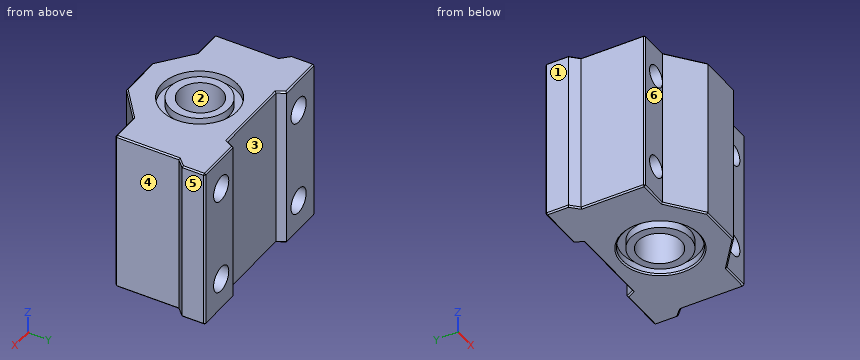
from build123d import *

# Parameters (mm, degrees)
SALIENTE_EXTRUIR1_DEPTH    = 15
CROQUIS2_R                 = 4
CORTAR_EXTRUIR1_DEPTH      = 37.239791666
CORTAR_EXTRUIR2_DEPTH      = 32.800786154
CORTAR_EXTRUIR2_DEPTH_BACK = 32.800786154
CROQUIS3_R                 = 2
SALIENTE_EXTRUIR2_DEPTH    = 30
CROQUIS5_R                 = 7
CROQUIS5_R_2               = 5.5
CORTAR_EXTRUIR3_DEPTH      = 1.5
CORTAR_EXTRUIR4_START      = -1.5
CROQUIS6_R                 = 7
CROQUIS6_R_2               = 5.5
CORTAR_EXTRUIR4_DEPTH      = 1.5
CROQUIS7_R                 = 2.35
CORTAR_EXTRUIR5_DEPTH      = 8.5
CHAFL_N1_SIZE              = 0.25


with BuildPart() as part:
    # Croquis1 → Saliente-Extruir1 (new, symmetric)
    with BuildSketch(Plane.XY):
        Polygon((-4, -11.15), (4, -11.15), (10, -6.35), (15.5, -6.35), (15.5, 5.4), (17, 6.9), (17, 11.15), (10, 11.15), (7.5, 9.65), (-7.5, 9.65), (-10, 11.15), (-17, 11.15), (-17, 6.9), (-15.5, 5.4), (-15.5, -6.35), (-10, -6.35), align=None)
    extrude(amount=SALIENTE_EXTRUIR1_DEPTH, both=True)

    # Croquis2 → Cortar-Extruir1 (cut, through all)
    with BuildSketch(Plane.XY.offset(15)):
        with Locations((0, 0.15)):
            Circle(CROQUIS2_R)
    extrude(amount=-CORTAR_EXTRUIR1_DEPTH, mode=Mode.SUBTRACT)

    # Croquis3 → Cortar-Extruir2 (cut, two sides: drawn at the far end of the back side and taken through both)
    with BuildSketch(Plane(origin=(0, 11.15, 0), x_dir=(1, 0, 0), z_dir=(0, 1, 0)).offset(-CORTAR_EXTRUIR2_DEPTH_BACK)):
        with Locations((-12, 9)):
            Circle(CROQUIS3_R)
        with Locations(Location((12, 9, 0), (0, 0, 180))):
            Circle(CROQUIS3_R)
        with Locations((-12, -9)):
            Circle(CROQUIS3_R)
        with Locations(Location((12, -9, 0), (0, 0, 180))):
            Circle(CROQUIS3_R)
    extrude(amount=CORTAR_EXTRUIR2_DEPTH + CORTAR_EXTRUIR2_DEPTH_BACK, mode=Mode.SUBTRACT)

    # Croquis4 → Saliente-Extruir2 (add, through all)
    with BuildSketch(Plane.XY.offset(15)):
        Polygon((-10, 11.15), (-7.5, 9.65), (-8.3, 11.15), align=None)
        Polygon((7.5, 9.65), (10, 11.15), (8.3, 11.15), align=None)
    extrude(amount=-SALIENTE_EXTRUIR2_DEPTH)

    # Croquis5 → Cortar-Extruir3 (cut)
    with BuildSketch(Plane.XY.offset(15)):
        Circle(CROQUIS5_R)
        Circle(CROQUIS5_R_2, mode=Mode.SUBTRACT)
    extrude(amount=-CORTAR_EXTRUIR3_DEPTH, mode=Mode.SUBTRACT)

    # Croquis6 → Cortar-Extruir4 (cut)
    with BuildSketch(Plane(origin=(0, 0, -15), x_dir=(-1, 0, 0), z_dir=(0, 0, -1)).offset(CORTAR_EXTRUIR4_START)):
        with Locations(Location((0, 0, 0), (0, 0, 180))):
            Circle(CROQUIS6_R)
        with Locations(Location((0, 0, 0), (0, 0, 180))):
            Circle(CROQUIS6_R_2, mode=Mode.SUBTRACT)
    extrude(amount=CORTAR_EXTRUIR4_DEPTH, mode=Mode.SUBTRACT)

    # Croquis7 → Cortar-Extruir5 (cut)
    with BuildSketch(Plane(origin=(0, 11.15, 0), x_dir=(1, 0, 0), z_dir=(0, 1, 0))):
        with Locations(Location((-12, 9, 0), (0, 0, 270))):
            Circle(CROQUIS7_R)
        with Locations(Location((-12, -9, 0), (0, 0, 270))):
            Circle(CROQUIS7_R)
        with Locations(Location((12, -9, 0), (0, 0, 270))):
            Circle(CROQUIS7_R)
        with Locations(Location((12, 9, 0), (0, 0, 270))):
            Circle(CROQUIS7_R)
    extrude(amount=-CORTAR_EXTRUIR5_DEPTH, mode=Mode.SUBTRACT)

    # Chaflán1
    chafl_n1_edges = [part.edges().sort_by_distance(p)[0] for p in [
        (0, 9.65, 15),
        (-7, 0, -15),
        (17, 9.025, -15),
        (16.25, 6.15, -15),
        (15.5, -0.475, -15),
        (12.75, -6.35, -15),
        (7, -8.75, -15),
        (-12.65, 11.15, 15),
        (0, -11.15, -15),
        (-7, -8.75, -15),
        (-12.75, -6.35, -15),
        (-15.5, -0.475, -15),
        (-16.25, 6.15, -15),
        (-17, 9.025, -15),
        (-12.65, 11.15, -15),
        (-17, 9.025, 15),
        (0, 9.65, -15),
        (12.65, 11.15, -15),
        (-16.25, 6.15, 15),
        (-15.5, -0.475, 15),
        (17, 11.15, 0),
        (15.5, -6.35, 0),
        (-15.5, -6.35, 0),
        (-17, 11.15, 0),
        (-12.75, -6.35, 15),
        (-7, -8.75, 15),
        (0, -11.15, 15),
        (7, -8.75, 15),
        (12.65, 11.15, 15),
        (12.75, -6.35, 15),
        (15.5, -0.475, 15),
        (16.25, 6.15, 15),
        (17, 9.025, 15),
        (-7.9, 10.4, -15),
        (-7.9, 10.4, 15),
        (7.9, 10.4, -15),
        (7.9, 10.4, 15),
    ]]
    chamfer(chafl_n1_edges, length=CHAFL_N1_SIZE)


solid = part.part
Work out the finished part from the listing and answer in its coordinate system (mm). Face numbers are marked on the shaded views. A direction names the side the tool comes from. Give positions to 0.01 mm unless a question says otherwise; leave off trailing zeros. Order: outer loops, then holes, each group sorted by start corner. A loop starts at its lowest first (then second) coordinate and runs counter-clockwise, first axis right, second up. Notation, with made-up numbers: (-2, -29.5) -> (49, -29.5) arc R7 ccw to (49, -18.5) -> close; hole circle Ø1 at (39, 41.25). An arc over 180 degrees is marked (long way). Answer as a JSON object with one key per item and string values. Group by question number.
1. Consider line 1 along Z through (x, y) = (-12, 0); line 2 along Y through (x, z) = (0, 14.65); line 3 along Z through (x, y) = (-13.5, 5.75). Determine where each line is inside the solid, lowest interval first. Write a range as [from, to].
2. Flat-ended cylindrical pins translate along their axes: pin 1 Ø6 at (x, z) = (12, 9) entering from -Y; pin 2 Ø1.5 at (x, z) = (8.5, 4.5) entering from -Y; pin 3 Ø10 at (y, z) = (6.5, -7.5) entering from -X; pin 4 Ø7.5 at (x, z) = (-12, -9) entering from -Y. Find the tip coordinate at first contact, or state that the pin passes through.
3. A tool of negligible diameter and unlimited length cuts with its end or side. For the marked faces 4, 5 and 6, from which of +Z, -Z, +X, -X, +Y, -Y can it reach the whole face along a straight path? Write none if from no direction.
4. The mould has two halves that part along Y. Classify the marked faces 1, 2 and 3: released by +Y, released by -Y, zero draft, split by the parting line, or undercut.
5. Section C-C on x = -12 is taken. Determine the outline of the cut face in (y, z), plus the area to 3 significant figures.
6. Section D-D on y = -2.75 is taken. Count the separate pieces of the cut face and the enclosed holes in it, plus the area to 3 significant figures.
7. Section B-B on z = 5.5 is taken. Determine the outline of the cut face in (x, y), plus the area to 3 significant figures.
Result sheet:
{
 "1": {"line 1": "z = [-15, -11], [-7, 7], [11, 15]", "line 2": "y = [-11.15, -7], [-5.5, -3.85], [4.15, 5.5], [7, 9.65]", "line 3": "z = [-15, -10.81], [-7.19, 7.19], [10.81, 15]"},
 "2": {"pin 1": "stops at y = -7.15", "pin 2": "stops at y = -8.15", "pin 3": "stops at x = -17", "pin 4": "stops at y = -7.75"},
 "3": {"face 4": "+Z, -Z, +X, -Y", "face 5": "+Z, -Z, +X, +Y, -Y", "face 6": "+Z, -Z, -X, -Y"},
 "4": {"face 1": "zero draft", "face 2": "undercut", "face 3": "released by +Y"},
 "5": {"outline": "(-6.35, -14.75) -> (-6.1, -15) -> (10.9, -15) -> (11.15, -14.75) -> (11.15, -11.35) -> (2.65, -11.35) -> (2.65, -11) -> (-6.35, -11) -> close; (-6.35, -7) -> (2.65, -7) -> (2.65, -6.65) -> (11.15, -6.65) -> (11.15, 6.65) -> (2.65, 6.65) -> (2.65, 7) -> (-6.35, 7) -> close; (-6.35, 11) -> (2.65, 11) -> (2.65, 11.35) -> (11.15, 11.35) -> (11.15, 14.75) -> (10.9, 15) -> (-6.1, 15) -> (-6.35, 14.75) -> close", "area": "373 mm^2"},
 "6": {"separate pieces": "2", "enclosed holes": "4", "area": "704 mm^2"},
 "7": {"outline": "(-17, 6.9) -> (-15.5, 5.4) -> (-15.5, -6.1) -> (-15.25, -6.35) -> (-10, -6.35) -> (-4, -11.15) -> (4, -11.15) -> (10, -6.35) -> (15.25, -6.35) -> (15.5, -6.1) -> (15.5, 5.4) -> (17, 6.9) -> (17, 10.9) -> (16.75, 11.15) -> (8.3, 11.15) -> (7.5, 9.65) -> (-7.5, 9.65) -> (-8.3, 11.15) -> (-16.75, 11.15) -> (-17, 10.9) -> close; hole circle Ø8 at (0, 0.15)", "area": "551 mm^2"}
}
